Verification items for the finished model (mm, model axes). A direction names the side the tool comes from. Coordinates: 2 decimals unless noted, no trailing zeros. Loops run counter-clockwise (first coordinate to the right, second up) from the corner with the lowest first, then second, coordinate; pieces in that order, holes last. Notation, with made-up numbers: (81, -11.75) -> (95, -11.75) arc R26 cw to (95, 12.25) -> close; hole circle Ø5 at (21.5, 17.5). An arc over 180 degrees is marked (long way). Answer as a JSON object with one key per item and string values. Group by question number.
Q1. Cross-section at C-C on x = 5. Record the boundary of the cut face in (y, z).
Q2. Scan lines: L1, parallel to X at y = 9.95, z = 2.5; L2, parallel to Z at x = -4.5, y = 11.5; L3, parallel to X at y = 11.75, z = 3.6. Record each from-to range of solid material in increasing order.
Q3. Cross-section at A-A on x = 0. Record the boundary of the cut face in (y, z).
Q4. Gauge pin test, flat end, axial feed: pin 1 Ø12 at (x, y) = (1, -2) entering from -Z. Record the tip position at first contact, or that the pin passes through.
Q5. Set-up check for faces 1 (the cylindrical face through (-2.11, -9.52, 3.03)), 2 (the flat face through (-9, 6, 5)), 3 (the cylindrical face through (5.69, 10.67, 2.88)): record each of +Z, -Z, +X, -X, +Y, -Y from which the full face is reachable in a straight line by a thin tool's end or side.
Q6. Cross-section at D-D on y = 8.5. Record the boundary of the cut face in (x, z), and give its area (3 significant figures).
Q7. Release check for a two-part mould opening along X. For faces 4 (the cylindrical face through (-5.75, 10.66, 2.55)), 5 (the flat face through (-9, 6, 0)), 6 (the flat face through (-12.5, 0, 2)) record: released by +X, released by -X, zero draft, split by the parting line, or undercut.
```python
from build123d import *

# Parameters (mm, degrees)
SKETCH1_W                 = 25
SKETCH1_H                 = 25
SKETCH1_R                 = 9.25
BOSS_EXTRUDE1_DEPTH       = 5
M3X0_5_TAPPED_HOLE1_D     = 2.5
M3X0_5_TAPPED_HOLE1_DEPTH = 7.5
M3X0_5_TAPPED_HOLE1_TIP   = 0.751075774
SKETCH4_R                 = 9.75
CUT_EXTRUDE1_DEPTH        = 4


with BuildPart() as part:
    # Sketch1 → Boss-Extrude1 (new body)
    with BuildSketch(Plane.XY):
        Rectangle(SKETCH1_W, SKETCH1_H)
        Circle(SKETCH1_R, mode=Mode.SUBTRACT)
    extrude(amount=BOSS_EXTRUDE1_DEPTH)

    # M3x0.5 Tapped Hole1
    with Locations(Plane(origin=(0, 12.5, 0), x_dir=(-1, 0, 0), z_dir=(0, 1, 0))):
        with Locations((4.5, 2.5), (-4.5, 2.5)):
            Hole(M3X0_5_TAPPED_HOLE1_D / 2, depth=M3X0_5_TAPPED_HOLE1_DEPTH)
            with Locations((0, 0, -(M3X0_5_TAPPED_HOLE1_DEPTH + M3X0_5_TAPPED_HOLE1_TIP / 2))):  # 118° drill point
                Cone(0, M3X0_5_TAPPED_HOLE1_D / 2, M3X0_5_TAPPED_HOLE1_TIP, mode=Mode.SUBTRACT)

    # Sketch4 → Cut-Extrude1 (cut)
    with BuildSketch(Plane.XY.offset(5)):
        Circle(SKETCH4_R)
    extrude(amount=-CUT_EXTRUDE1_DEPTH, mode=Mode.SUBTRACT)


solid = part.part
```
Computed values:
{
 "1": {"outline": "(-12.5, 0) -> (-7.78, 0) -> (-7.78, 1) -> (-8.37, 1) -> (-8.37, 5) -> (-12.5, 5) -> close; (7.78, 0) -> (12.5, 0) -> (12.5, 1.35) -> (8.37, 1.35) -> (8.37, 1) -> (7.78, 1) -> close; (8.37, 3.65) -> (12.5, 3.65) -> (12.5, 5) -> (8.37, 5) -> close"},
 "2": {"L1": "x = -12.5 to -5.75, -3.25 to 3.25, 5.75 to 12.5", "L2": "z = 0 to 1.25, 3.75 to 5", "L3": "x = -12.5 to -5.09, -3.91 to 3.91, 5.09 to 12.5"},
 "3": {"outline": "(-12.5, 0) -> (-9.25, 0) -> (-9.25, 1) -> (-9.75, 1) -> (-9.75, 5) -> (-12.5, 5) -> close; (9.25, 0) -> (12.5, 0) -> (12.5, 5) -> (9.75, 5) -> (9.75, 1) -> (9.25, 1) -> close"},
 "4": {"pin 1": "passes through"},
 "5": {"face 1": "+Z", "face 2": "+Z, +X, -X, +Y, -Y", "face 3": "+Y"},
 "6": {"outline": "(-12.5, 0) -> (-3.65, 0) -> (-3.65, 1) -> (-4.78, 1) -> (-4.78, 1.28) arc R1.25 cw to (-4.78, 3.72) -> (-4.78, 5) -> (-12.5, 5) -> close; (3.65, 0) -> (12.5, 0) -> (12.5, 5) -> (4.78, 5) -> (4.78, 3.72) arc R1.25 cw to (4.78, 1.28) -> (4.78, 1) -> (3.65, 1) -> close", "area": "76.0 mm²"},
 "7": {"face 4": "undercut", "face 5": "zero draft", "face 6": "released by -X"}
}
